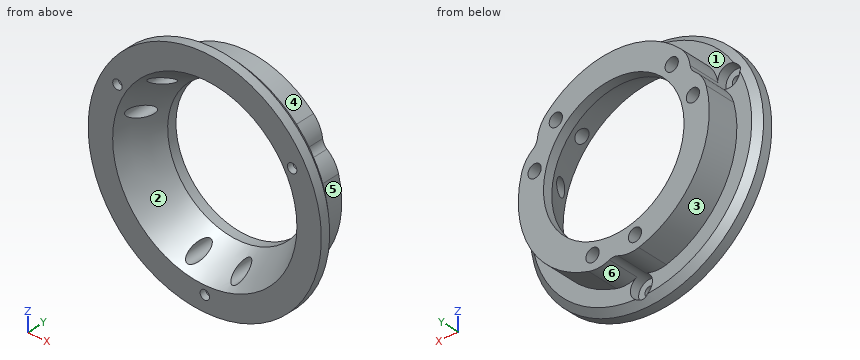
from build123d import *

# Parameters (mm, degrees)
SKETCH1_R           = 30.3
SKETCH1_R_2         = 22.3
BOSS_EXTRUDE1_DEPTH = 10
BOSS_EXTRUDE2_START = -5
SKETCH2_R           = 37
SKETCH2_R_2         = 22.3
BOSS_EXTRUDE2_DEPTH = 5
SKETCH3_R           = 1.5
CUT_EXTRUDE1_DEPTH  = 54.272882407
CUT_EXTRUDE2_START  = -3
SKETCH4_R           = 3.5
CUT_EXTRUDE2_DEPTH  = 57.272882407
CIRPATTERN1_COUNT   = 3
CHAMFER1_SIZE       = 12
CHAMFER1_SIZE2      = 6.92820323
CHAMFER2_SIZE       = 2
SKETCH5_R           = 2.1
CUT_EXTRUDE3_DEPTH  = 55.433445737
CIRPATTERN2_COUNT   = 3
FILLET1_R           = 10


with BuildPart() as part:
    # Sketch1 → Boss-Extrude1 (new body)
    with BuildSketch(Plane(origin=(0, 0, 0), x_dir=(1, 0, 0), z_dir=(0, 1, 0))):
        with Locations(Location((0, 0, 0), (0, 0, 270))):
            Circle(SKETCH1_R)
        with Locations(Location((0, 0, 0), (0, 0, 270))):
            Circle(SKETCH1_R_2, mode=Mode.SUBTRACT)
    extrude(amount=BOSS_EXTRUDE1_DEPTH)

    # Sketch2 → Boss-Extrude2 (add)
    with BuildSketch(Plane(origin=(0, 0, 0), x_dir=(1, 0, 0), z_dir=(0, 1, 0)).offset(BOSS_EXTRUDE2_START)):
        with Locations(Location((0, 0, 0), (0, 0, 270))):
            Circle(SKETCH2_R)
        with Locations(Location((0, 0, 0), (0, 0, 270))):
            Circle(SKETCH2_R_2, mode=Mode.SUBTRACT)
    extrude(amount=BOSS_EXTRUDE2_DEPTH)

    # Sketch3 → Cut-Extrude1 (cut, through all)
    with BuildSketch(Plane(origin=(0, 0, 0), x_dir=(1, 0, 0), z_dir=(0, 1, 0))):
        with Locations(Location((0, 32, 0), (0, 0, 270))):
            Circle(SKETCH3_R)
    cut_extrude1 = extrude(amount=-CUT_EXTRUDE1_DEPTH, mode=Mode.SUBTRACT)

    # Sketch4 → Cut-Extrude2 (cut)
    with BuildSketch(Plane(origin=(0, 0, 0), x_dir=(1, 0, 0), z_dir=(0, 1, 0)).offset(CUT_EXTRUDE2_START)):
        with Locations(Location((0, 32, 0), (0, 0, 328.163304996))):
            Circle(SKETCH4_R)
    cut_extrude2 = extrude(amount=CUT_EXTRUDE2_DEPTH, mode=Mode.SUBTRACT)

    # CirPattern1: Cut-Extrude1, Cut-Extrude2 ×3 about axis
    cirpattern1_axis = Axis((0, 0, 0), (0, 1, 0))
    add([cut_extrude1.rotate(cirpattern1_axis, i * 360 / CIRPATTERN1_COUNT) for i in range(1, CIRPATTERN1_COUNT)], mode=Mode.SUBTRACT)
    add([cut_extrude2.rotate(cirpattern1_axis, i * 360 / CIRPATTERN1_COUNT) for i in range(1, CIRPATTERN1_COUNT)], mode=Mode.SUBTRACT)

    # Chamfer1
    chamfer1_edges = [part.edges().sort_by_distance(p)[0] for p in [
        (0, -5, -22.3),
    ]]
    chamfer1_side = [part.faces().sort_by_distance(p)[0] for p in [
        (0, 2.5, -22.3),
    ]]
    chamfer(chamfer1_edges, length=CHAMFER1_SIZE, length2=CHAMFER1_SIZE2, reference=chamfer1_side[0])

    # Chamfer2
    # the kernel refuses this chamfer: 2 mm, written as the material it takes off along each edge
    with BuildSketch(Plane(origin=(0, 0, 0), x_dir=(0, 0, 1), z_dir=(-1, 0, 0))) as chamfer2_piece_1:
        Polygon((37, -CHAMFER2_SIZE), (37 - CHAMFER2_SIZE, 0), (37, 0), align=None)
    revolve(axis=Axis((0, 0, 0), (0, 1, 0)), mode=Mode.SUBTRACT)

    # Sketch5 → Cut-Extrude3 (cut, through all)
    with BuildSketch(Plane(origin=(0, 10, 0), x_dir=(1, 0, 0), z_dir=(0, 1, 0))):
        with Locations(Location((6.729295173, 25.114071484, 0), (0, 0, 270))):
            Circle(SKETCH5_R)
        with Locations(Location((-6.729295173, 25.114071484, 0), (0, 0, 270))):
            Circle(SKETCH5_R)
    cut_extrude3 = extrude(amount=-CUT_EXTRUDE3_DEPTH, mode=Mode.SUBTRACT)

    # CirPattern2: Cut-Extrude3 ×3 about axis
    cirpattern2_axis = Axis((0, 0, 0), (0, 1, 0))
    for i in range(1, CIRPATTERN2_COUNT):
        add(cut_extrude3.rotate(cirpattern2_axis, i * 360 / CIRPATTERN2_COUNT), mode=Mode.SUBTRACT)

    # Fillet1
    # the kernel refuses this fillet: 10 mm, written as the material it takes off along each edge
    with BuildSketch(Plane(origin=(2.973442607, 0, -30.15375), x_dir=(0.9835455418768547, 0, 0.18066036381609613), z_dir=(0, 1, 0)), Plane(origin=(-27.600634823, 0, 12.501798166), x_dir=(-0.33531630641674726, 0, -0.9421056069523365), z_dir=(0, 1, 0)), Plane(origin=(-24.627192216, 22.615356127, 17.651951834), x_dir=(0.6482292354635445, 0, 0.7614452431333121), z_dir=(0, -1, 0)), Plane(origin=(27.600634823, 22.615356127, 12.501798166), x_dir=(0.33531630641249444, 0, -0.9421056069538499), z_dir=(0, -1, 0))) as fillet1_piece_1:
        with BuildLine():
            CenterArc((4.213445677, -9.965270497), FILLET1_R, 85.223468089, 38.380201644)
            ThreePointArc((-1.321003282, -1.636412549), (-0.534685103, -0.919772386), (0, 0))
            ThreePointArc((0, 0), (2.523071225, 0.105230393), (5.046142451, 0))
        make_face()
    extrude(amount=22.615356127, mode=Mode.SUBTRACT)
    with BuildSketch(Plane(origin=(-2.973442607, 22.615356127, -30.15375), x_dir=(0.758369035624482, 0, 0.6518254412079917), z_dir=(0, -1, 0)), Plane(origin=(24.627192216, 0, 17.651951834), x_dir=(-0.18531287310344324, 0, -0.9826795708989514), z_dir=(0, 1, 0))) as fillet1_piece_2:
        with BuildLine():
            CenterArc((5.107451253, 9.538012489), FILLET1_R, 214.135867483, 38.380201644)
            ThreePointArc((-3.169640839, 3.926439938), (-1.66670095, 1.897121448), (0, 0))
            ThreePointArc((0, 0), (1.051534082, 0.161695629), (2.103068163, 0))
        make_face()
    extrude(amount=22.615356127, mode=Mode.SUBTRACT)


solid = part.part
Design review of the part built by this model. Coordinates are the model's own, in mm. Face numbers are marked on the shaded views. A direction names the side the tool comes from. Coordinates: 2 decimals unless noted, no trailing zeros. Loops run counter-clockwise (first coordinate to the right, second up) from the corner with the lowest first, then second, coordinate; pieces in that order, holes last. Notation, with made-up numbers: (14.5, 80.5) -> (31.5, 80.5) arc R20 cw to (31.5, 103.5) -> close; hole circle Ø11 at (-27.75, -29). An arc over 180 degrees is marked (long way). Use a Markdown table: item, result. Add a question column.
Item 1: The part is to be moulded in two halves that separate along Z. For the marked faces 1, 2 and 3, say which applies: +Z half, -Z half, draft (parallel to the pull), parting line (faces both ways), or undercut.
Item 2: Machinability: for the marked faces 4, 5 and 6, which of the approach directions +Z, -Z, +X, -X, +Y, -Y give a long, thin tool a straight path to every point of the face, cutting with its end or side? Answer none if there is none.
Item 3: Clearance check with flat-ended pins moving along their axes: P1, Ø6.5, axis at x = -6.73, z = -25.11, coming from the +Y side; P2, Ø2, axis at x = -0.5, z = -32.5, coming from the +Y side; P3, Ø5, axis at x = 18.38, z = 18.38, coming from the -Y side; P4, Ø5, axis at x = -5, y = 3.5, coming from the -Z side. State where each tip first meets the part, or that it passes through.
Item 4: We need section A-A, the plane x = 0. Write out the cut boundary in (y, z), and give its area (3 significant figures).
Item 5: We need section C-C, the plane z = -25. Count the separate pieces of the cut face and the enclosed holes in it, and give its area (3 significant figures).
Item 6: We need section B-B, the plane z = 0. Write out the cut boundary in (x, y), and give its area (3 significant figures).
Item 7: Wall thickness on L1, parallel to Z at x = -1, y = -1.5; L2, parallel to X at y = 8.8, z = 0; L3, parallel to X at y = 6.5, z = -27: over which ranges is each line inside the solid? List them lowest first. Write a range as from..to.
Numbers:
| question | item | result |
|---|---|---|
| 1 | face 1 | draft |
| 1 | face 2 | undercut |
| 1 | face 3 | parting line |
| 2 | face 4 | +Z, +Y |
| 2 | face 5 | +X, +Y |
| 2 | face 6 | -Z, +Y |
| 3 | P1 | stops at y = 10 |
| 3 | P2 | stops at y = -3 |
| 3 | P3 | stops at y = -3.73 |
| 3 | P4 | stops at z = -29.59 |
| 4 | outline | (-5, -37) -> (-2, -37) -> (-0.5, -35.5) -> (-3, -35.5) -> (-3, -33.5) -> (-5, -33.5) -> close; (-5, -30.5) -> (-3, -30.5) -> (-3, -28.5) -> (10, -28.5) -> (10, -22.3) -> (7, -22.3) -> (-5, -29.23) -> close; (-5, 29.23) -> (7, 22.3) -> (10, 22.3) -> (10, 30.3) -> (0, 30.3) -> (0, 35) -> (-2, 37) -> (-5, 37) -> close |
| 4 | area | 175 mm^2 |
| 5 | separate pieces | 3 |
| 5 | enclosed holes | 0 |
| 5 | area | 386 mm^2 |
| 6 | outline | (-37, -5) -> (-29.23, -5) -> (-22.3, 7) -> (-22.3, 10) -> (-30.3, 10) -> (-30.3, 0) -> (-35, 0) -> (-37, -2) -> close; (22.3, 7) -> (29.23, -5) -> (37, -5) -> (37, -2) -> (35, 0) -> (30.3, 0) -> (30.3, 10) -> (22.3, 10) -> close |
| 6 | area | 220 mm^2 |
| 7 | L1 | z = -36.49..-35.35, -28.65..-27.19, 27.19..36.49 |
| 7 | L2 | x = -30.3..-22.3, 22.3..30.3 |
| 7 | L3 | x = -13.75..-7.65, -5.81..5.81, 7.65..13.75 |
